Geometry: see drawing. Coordinates: mm, zero at the bounding-box minimum. Round coordinates to 2 decimals unless told otherwise and drop trailing zeros. Write each loop counter-clockwise with the first axis right and the second up, starting at its lowest first coordinate (ties: lowest second). Pieces come first, ordered by that corner, then holes. Notation, with made-up numbers: M -34,-11.5 L -7,-11.5 A25 ccw -7,13.5 Z; hole C 56.25,-7.5 d2. An arc over 180 degrees is marked long. Use one line per item in the form item = value. Start each with the question number.
Item 1: Ray query, probe 1 along Z at (x, y) = (63.5, 2.9); probe 2 along X at (y, z) = (4.65, 42.5); probe 3 along Z at (x, y) = (60, 1.7). Return the intervals inside material, ascending.
Item 2: Section query B-B (y = 1.4). Return loops of the section in (x, z), and give its area (3 significant figures).
Item 3: Section query A-A (x = 63.5). Return loops of the section in (y, z).
Item 4: Section query D-D (x = 38.5). Return loops of the section in (y, z), and give its area (3 significant figures).
Item 5: Section query C-C (z = 266.7). Return loops of the section in (x, y).
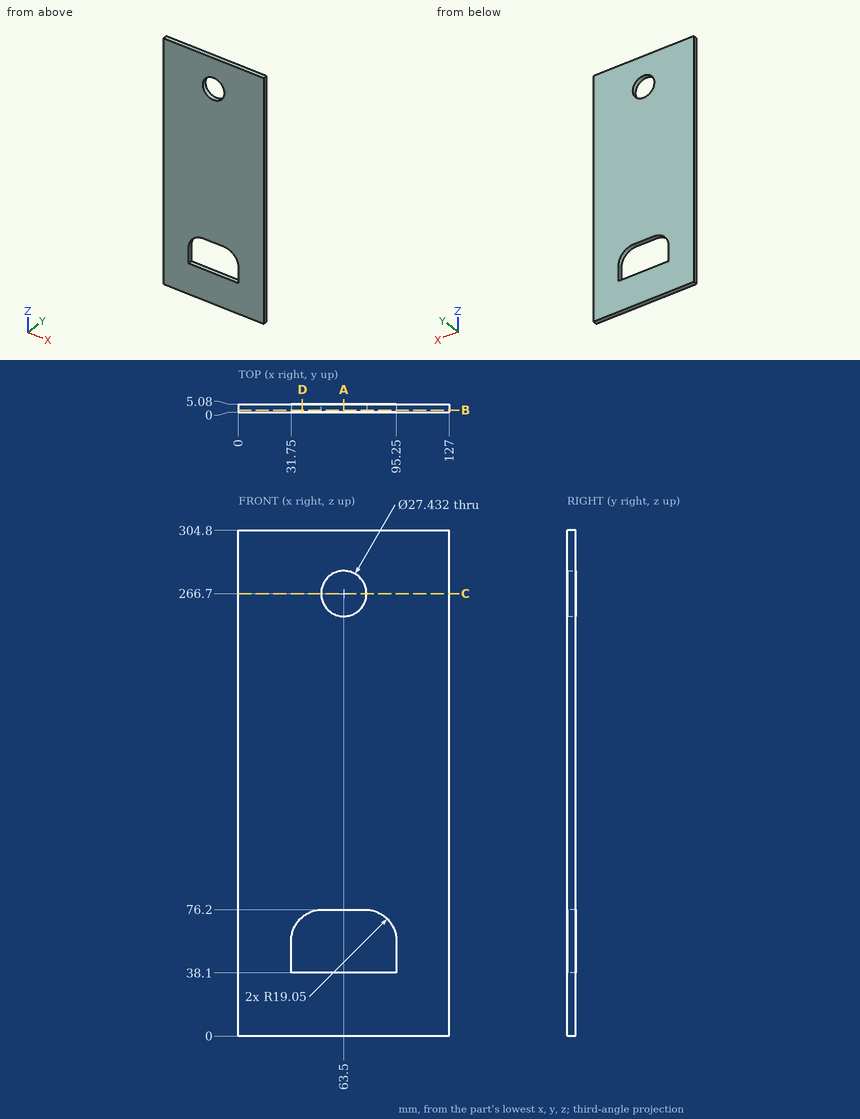
Working result:
q1.probe_1 = 0 to 38.1, 76.2 to 252.98, 280.42 to 304.8
q1.probe_2 = 0 to 31.75, 95.25 to 127
q1.probe_3 = 0 to 38.1, 76.2 to 253.44, 279.96 to 304.8
q2.outline = M 0,0 L 127,0 L 127,304.8 L 0,304.8 Z; hole M 31.75,38.1 L 95.25,38.1 L 95.25,57.15 A19.05 ccw 76.2,76.2 L 50.8,76.2 A19.05 ccw 31.75,57.15 Z; hole C 63.5,266.7 d27.43
q2.area = 35,900 mm²
q3.outline = M 0,0 L 5.08,0 L 5.08,38.1 L 0,38.1 Z; M 0,76.2 L 5.08,76.2 L 5.08,252.98 L 0,252.98 Z; M 0,280.42 L 5.08,280.42 L 5.08,304.8 L 0,304.8 Z
q4.outline = M 0,0 L 5.08,0 L 5.08,38.1 L 0,38.1 Z; M 0,71.7 L 5.08,71.7 L 5.08,304.8 L 0,304.8 Z
q4.area = 1,380 mm²
q5.outline = M 0,0 L 49.78,0 L 49.78,5.08 L 0,5.08 Z; M 77.22,0 L 127,0 L 127,5.08 L 77.22,5.08 Z
